Check sheet for the drawn part. Datum: minimum x, y, z corner. Units: mm. A direction names the side the tool comes from. Coordinates: 2 decimals unless noted, no trailing zeros. Order: outer loops, then holes, each group sorted by start corner. A loop starts at its lowest first (then second) coordinate and runs counter-clockwise, first axis right, second up.
Q1. Cross-section at B-B, the plane z = 10.5. Record the boundary of the cut face in (x, y).
Q2. Set-up check for the marked faces 5, 6, 7 and 8: record each of +Z, -Z, +X, -X, +Y, -Y from which the full face is reachable in a straight line by a thin tool's end or side.
Q3. Thickness scan on line 1 (X direction, y = 34, z = 25.5); line 2 (Z direction, x = 73.5, y = 68.5); line 3 (Z direction, x = 128.5, y = 50.5). Record the ranges inside material, lowest first.
Q4. Cross-section at D-D, the plane y = 60.5. Record the boundary of the cut face in (x, z).
Q5. Cross-section at A-A, the plane x = 83. Record the boundary of the cut face in (y, z).
Q6. Cross-section at C-C, the plane y = 38.5. Record the boundary of the cut face in (x, z), and give its area (3 significant figures).
Q7. Draft check along X on the marked faces 1, 2, 3 and 4. Enter one of: pulls with the +X half, pulls with the -X half, needs draft (parallel to the pull), parting line crosses it, or undercut.
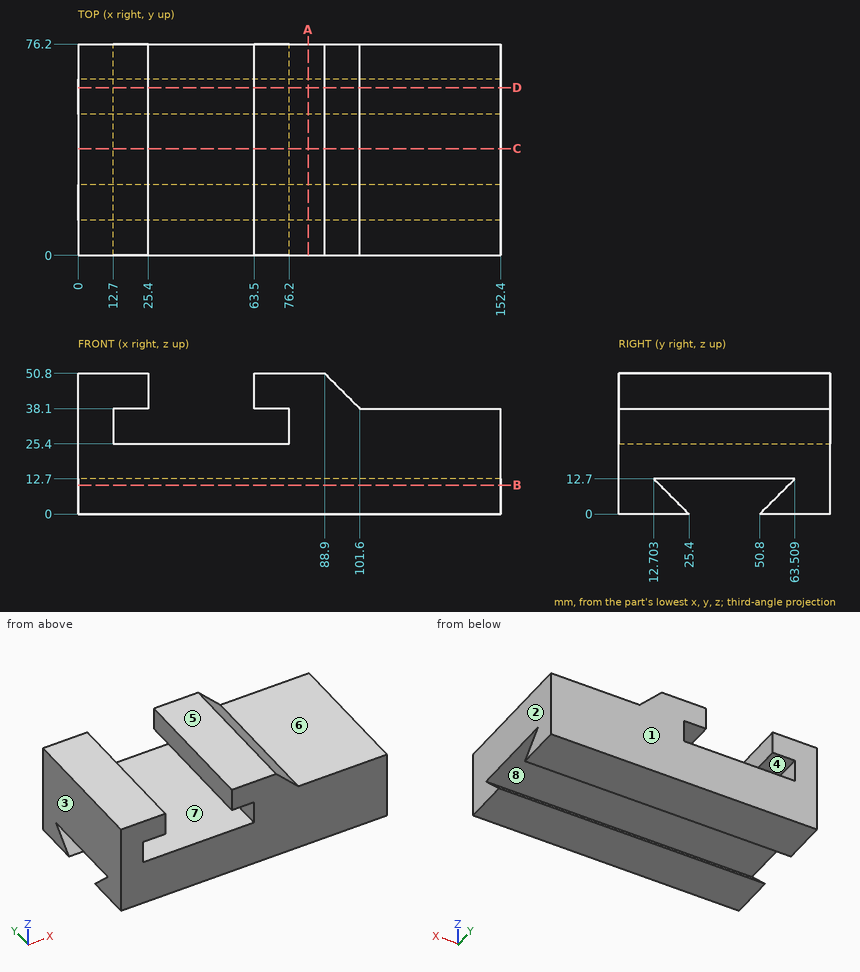
Check values:
1. outline: (0, 0) - (152.4, 0) - (152.4, 14.9) - (0, 14.9) - close; (0, 61.31) - (152.4, 61.31) - (152.4, 76.2) - (0, 76.2) - close
2. face 5: +Z, +X, -X, +Y, -Y
2. face 6: +Z, +X, +Y, -Y
2. face 7: +Y, -Y
2. face 8: +X, -X
3. line 1: x = 0 to 12.7, 76.2 to 152.4
3. line 2: z = 0 to 25.4, 38.1 to 50.8
3. line 3: z = 12.7 to 38.1
4. outline: (0, 0) - (152.4, 0) - (152.4, 9.69) - (0, 9.69) - close; (0, 12.7) - (152.4, 12.7) - (152.4, 38.1) - (101.6, 38.1) - (88.9, 50.8) - (63.5, 50.8) - (63.5, 38.1) - (76.2, 38.1) - (76.2, 25.4) - (12.7, 25.4) - (12.7, 38.1) - (25.4, 38.1) - (25.4, 50.8) - (0, 50.8) - close
5. outline: (0, 0) - (25.4, 0) - (12.7, 12.7) - (63.51, 12.7) - (50.8, 0) - (76.2, 0) - (76.2, 50.8) - (0, 50.8) - close
6. outline: (0, 12.7) - (152.4, 12.7) - (152.4, 38.1) - (101.6, 38.1) - (88.9, 50.8) - (63.5, 50.8) - (63.5, 38.1) - (76.2, 38.1) - (76.2, 25.4) - (12.7, 25.4) - (12.7, 38.1) - (25.4, 38.1) - (25.4, 50.8) - (0, 50.8) - close
6. area: 3,790 mm2
7. face 1: needs draft
7. face 2: pulls with the +X half
7. face 3: pulls with the -X half
7. face 4: undercut
